Could you check a few things on this model? Use its own coordinates, in mm. Give positions to 0.01 mm unless a question says otherwise; leave off trailing zeros. Order: outer loops, then holes, each group sorted by start corner. A loop starts at its lowest first (then second) coordinate and runs counter-clockwise, first axis right, second up. Notation, with made-up numbers: (78, 53) - (100, 53) arc R7 cw to (100, 64) - close; hole circle Ø2 at (6, -20.5). An arc over 180 degrees is marked (long way). One line per question, with ' | ' between items. Start each with the question number.
1. Imagine slicing it at C-C (y = 5.25). Please give me the cut outline in (x, z), and give its area (3 significant figures).
2. If we mould it in two halves opening along X, with no side actions, what happens to faces 1 (the cylindrical face through (1.233, 9.735, -125.724)), 2 (the flat face through (1, 12.954, -133)), 3 (the cylindrical face through (8.61, 20.66, -133.64))? For each: released by +X, released by -X, zero draft, split by the parting line, or undercut.
3. I need wall thicknesses on probe 1 along Y at (x, z) = (-6.75, -131.5); probe 2 along X at (y, z) = (16.25, -135.25); probe 3 along Z at (x, y) = (11.75, 9.75). Which ranges of each line are inside material? Lowest first, please. Write a range as from..to.
4. For P1, Ø6, axis at y = 25, z = -128.5, coming from the -X side; P2, Ø4, axis at x = 7.5, z = -137.5, coming from the -Y side; P3, Ø6, axis at x = -2, y = 11, coming from the +Z side, each with a flat end and sliding along its axis, tell me the tip position at first contact or that it passes through.
5. Imagine slicing it at A-A (y = 12). Please give me the cut outline in (x, z), and give its area (3 significant figures).
6. Imagine slicing it at B-B (y = 21.75). Please give me the cut outline in (x, z).
```python
from build123d import *

# Parameters (mm, degrees)
SKETCH1_R           = 140.97
SKETCH1_R_2         = 125.73
BOSS_EXTRUDE1_DEPTH = 12.954
CUT_EXTRUDE1_START  = -12.954
CUT_EXTRUDE1_DEPTH  = 12.954
SKETCH5_R           = 2.1209
BOSS_EXTRUDE2_DEPTH = 28.575
SKETCH6_W           = 35.941656598
SKETCH6_H           = 50
CUT_EXTRUDE2_DEPTH  = 25.4


with BuildPart() as part:
    # Sketch1 → Boss-Extrude1 (new body)
    with BuildSketch(Plane(origin=(0, 0, 0), x_dir=(1, 0, 0), z_dir=(0, 1, 0))):
        with Locations(Location((0, 0, 0), (0, 0, 270))):
            Circle(SKETCH1_R)
        with Locations(Location((0, 0, 0), (0, 0, 270))):
            Circle(SKETCH1_R_2, mode=Mode.SUBTRACT)
    extrude(amount=BOSS_EXTRUDE1_DEPTH)

    # Sketch3 → Cut-Extrude1 (cut)
    with BuildSketch(Plane(origin=(0, 12.954, 0), x_dir=(1, 0, 0), z_dir=(0, 1, 0)).offset(CUT_EXTRUDE1_START)):
        with BuildLine():
            Line((13.491584054, 140.322906397), (12.033034426, 125.152862462))
            ThreePointArc((12.033034426, 125.152862462), (93.061663209, 84.54324184), (125.73, 0))
            ThreePointArc((125.73, 0), (-85.339106447, -92.332387659), (-9.882340901, 125.341023764))
            Line((-9.882340901, 125.341023764), (-11.080200404, 140.53387513))
            ThreePointArc((-11.080200404, 140.53387513), (-95.683240562, -103.524192223), (140.97, 0))
            ThreePointArc((140.97, 0), (104.34186481, 94.790907517), (13.491584054, 140.322906397))
        make_face()
    extrude(amount=CUT_EXTRUDE1_DEPTH, mode=Mode.SUBTRACT)

    # Sketch5 → Boss-Extrude2 (add)
    with BuildSketch(Plane(origin=(0, 0, 0), x_dir=(1, 0, 0), z_dir=(0, 1, 0))):
        with Locations(Location((10.71230924, 133.345085246, 0), (0, 0, 2.80489485))):
            Circle(SKETCH5_R)
    extrude(amount=BOSS_EXTRUDE2_DEPTH)

    # Sketch2 → Cut-Revolve1 (revolve, cut)
    with BuildSketch(Plane.XY):
        with BuildLine():
            Line((-125.73, 6.604), (-125.73, 0))
            Line((-125.73, 0), (-140.97, 0))
            ThreePointArc((-140.97, 0), (-133.78949329, 4.316215284), (-125.73, 6.604))
        make_face()
    revolve(axis=Axis((0, 0, 0), (0, 1, 0)), mode=Mode.SUBTRACT)

    # Sketch6 → Cut-Extrude2 (cut)
    with BuildSketch(Plane(origin=(0, 0, 0), x_dir=(0.09570535612916914, 0, -0.9954097070092239), z_dir=(0.995409707009224, 0, 0.09570535612916914))):
        with Locations((132.91957607, 23.563430101)):
            Rectangle(SKETCH6_W, SKETCH6_H)
    extrude(amount=CUT_EXTRUDE2_DEPTH, mode=Mode.SUBTRACT)


solid = part.part
```
Results found:
1) outline: (-11.08, -140.53) arc R140.97 ccw to (13.49, -140.32) - (12.57, -130.76) arc R131.37 cw to (-10.33, -130.96) - close | area: 228 mm2
2) face 1: undercut | face 2: zero draft | face 3: split by the parting line
3) probe 1: y = 5.14..12.95 | probe 2: x = 9.78..11.64 | probe 3: z = -140.48..-125.18
4) P1: stops at x = 9.67 | P2: stops at y = 0.96 | P3: stops at z = -125.63
5) outline: (-11.08, -140.53) arc R140.97 ccw to (13.49, -140.32) - (12.03, -125.15) arc R125.73 cw to (-9.88, -125.34) - close | area: 355 mm2
6) outline: (12.77, -132.84) arc R2.12 ccw (long way) to (12.83, -133.45) - close
